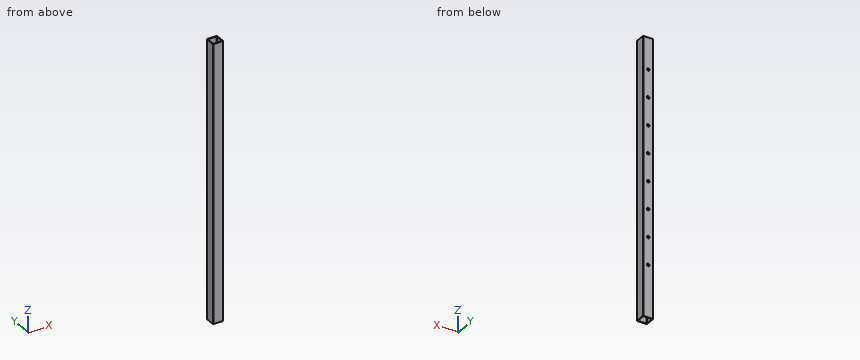
from build123d import *

# Parameters (mm, degrees)
SKETCH3_W           = 19.05
SKETCH3_H           = 19.05
SKETCH3_W_2         = 16.5608
SKETCH3_H_2         = 16.5608
BOSS_EXTRUDE1_DEPTH = 254.635
FILLET1_R           = 1.2446
CUT_EXTRUDE1_REACH  = 257.524
SKETCH4_R           = 2.413


with BuildPart() as part:
    # Sketch3 → Boss-Extrude1 (new, symmetric)
    with BuildSketch(Plane.XY):
        Rectangle(SKETCH3_W, SKETCH3_H)
        Rectangle(SKETCH3_W_2, SKETCH3_H_2, mode=Mode.SUBTRACT)
    extrude(amount=BOSS_EXTRUDE1_DEPTH, both=True)

    # Fillet1
    fillet1_edges = [part.edges().sort_by_distance(p)[0] for p in [
        (-8.2804, -8.2804, 0),
        (8.2804, -8.2804, 0),
        (8.2804, 8.2804, 0),
        (-8.2804, 8.2804, 0),
        (9.525, -9.525, 0),
        (-9.525, -9.525, 0),
        (-9.525, 9.525, 0),
        (9.525, 9.525, 0),
    ]]
    fillet(fillet1_edges, radius=FILLET1_R)

    # Sketch4 → Cut-Extrude1 (cut, up to next)
    with BuildSketch(Plane(origin=(0, 9.525, 0), x_dir=(1, 0, 0), z_dir=(0, 1, 0)), mode=Mode.PRIVATE) as cut_extrude1_sk1:
        with Locations(Location((0, 159.385, 0), (0, 0, 270))):
            Circle(SKETCH4_R)
    cut_extrude1_tool1 = extrude(cut_extrude1_sk1.sketch, amount=-CUT_EXTRUDE1_REACH, mode=Mode.PRIVATE) & part.part
    # Sketch4 → Cut-Extrude1 (cut, up to next)
    with BuildSketch(Plane(origin=(0, 9.525, 0), x_dir=(1, 0, 0), z_dir=(0, 1, 0)), mode=Mode.PRIVATE) as cut_extrude1_sk2:
        with Locations(Location((0, 108.585, 0), (0, 0, 270))):
            Circle(SKETCH4_R)
    cut_extrude1_tool2 = extrude(cut_extrude1_sk2.sketch, amount=-CUT_EXTRUDE1_REACH, mode=Mode.PRIVATE) & part.part
    # Sketch4 → Cut-Extrude1 (cut, up to next)
    with BuildSketch(Plane(origin=(0, 9.525, 0), x_dir=(1, 0, 0), z_dir=(0, 1, 0)), mode=Mode.PRIVATE) as cut_extrude1_sk3:
        with Locations(Location((0, 57.785, 0), (0, 0, 270))):
            Circle(SKETCH4_R)
    cut_extrude1_tool3 = extrude(cut_extrude1_sk3.sketch, amount=-CUT_EXTRUDE1_REACH, mode=Mode.PRIVATE) & part.part
    # Sketch4 → Cut-Extrude1 (cut, up to next)
    with BuildSketch(Plane(origin=(0, 9.525, 0), x_dir=(1, 0, 0), z_dir=(0, 1, 0)), mode=Mode.PRIVATE) as cut_extrude1_sk4:
        with Locations(Location((0, 6.985, 0), (0, 0, 270))):
            Circle(SKETCH4_R)
    cut_extrude1_tool4 = extrude(cut_extrude1_sk4.sketch, amount=-CUT_EXTRUDE1_REACH, mode=Mode.PRIVATE) & part.part
    # Sketch4 → Cut-Extrude1 (cut, up to next)
    with BuildSketch(Plane(origin=(0, 9.525, 0), x_dir=(1, 0, 0), z_dir=(0, 1, 0)), mode=Mode.PRIVATE) as cut_extrude1_sk5:
        with Locations(Location((0, -43.815, 0), (0, 0, 270))):
            Circle(SKETCH4_R)
    cut_extrude1_tool5 = extrude(cut_extrude1_sk5.sketch, amount=-CUT_EXTRUDE1_REACH, mode=Mode.PRIVATE) & part.part
    # Sketch4 → Cut-Extrude1 (cut, up to next)
    with BuildSketch(Plane(origin=(0, 9.525, 0), x_dir=(1, 0, 0), z_dir=(0, 1, 0)), mode=Mode.PRIVATE) as cut_extrude1_sk6:
        with Locations(Location((0, -94.615, 0), (0, 0, 270))):
            Circle(SKETCH4_R)
    cut_extrude1_tool6 = extrude(cut_extrude1_sk6.sketch, amount=-CUT_EXTRUDE1_REACH, mode=Mode.PRIVATE) & part.part
    # Sketch4 → Cut-Extrude1 (cut, up to next)
    with BuildSketch(Plane(origin=(0, 9.525, 0), x_dir=(1, 0, 0), z_dir=(0, 1, 0)), mode=Mode.PRIVATE) as cut_extrude1_sk7:
        with Locations(Location((0, -145.415, 0), (0, 0, 270))):
            Circle(SKETCH4_R)
    cut_extrude1_tool7 = extrude(cut_extrude1_sk7.sketch, amount=-CUT_EXTRUDE1_REACH, mode=Mode.PRIVATE) & part.part
    # Sketch4 → Cut-Extrude1 (cut, up to next)
    with BuildSketch(Plane(origin=(0, 9.525, 0), x_dir=(1, 0, 0), z_dir=(0, 1, 0)), mode=Mode.PRIVATE) as cut_extrude1_sk8:
        with Locations(Location((0, -196.215, 0), (0, 0, 270))):
            Circle(SKETCH4_R)
    cut_extrude1_tool8 = extrude(cut_extrude1_sk8.sketch, amount=-CUT_EXTRUDE1_REACH, mode=Mode.PRIVATE) & part.part
    add(cut_extrude1_tool1.solids().sort_by_distance((0, 9.525, -159.385))[0], mode=Mode.SUBTRACT)
    add(cut_extrude1_tool2.solids().sort_by_distance((0, 9.525, -108.585))[0], mode=Mode.SUBTRACT)
    add(cut_extrude1_tool3.solids().sort_by_distance((0, 9.525, -57.785))[0], mode=Mode.SUBTRACT)
    add(cut_extrude1_tool4.solids().sort_by_distance((0, 9.525, -6.985))[0], mode=Mode.SUBTRACT)
    add(cut_extrude1_tool5.solids().sort_by_distance((0, 9.525, 43.815))[0], mode=Mode.SUBTRACT)
    add(cut_extrude1_tool6.solids().sort_by_distance((0, 9.525, 94.615))[0], mode=Mode.SUBTRACT)
    add(cut_extrude1_tool7.solids().sort_by_distance((0, 9.525, 145.415))[0], mode=Mode.SUBTRACT)
    add(cut_extrude1_tool8.solids().sort_by_distance((0, 9.525, 196.215))[0], mode=Mode.SUBTRACT)


solid = part.part
CAD build for the part. Positions are in the model's coordinates, mm. Round coordinates to 2 decimals unless told otherwise and drop trailing zeros. Write each loop counter-clockwise with the first axis right and the second up, starting at its lowest first coordinate (ties: lowest second). Pieces come first, ordered by that corner, then holes. Notation, with made-up numbers: M 57.5,65.25 L 107.5,65.25 A29 cw 107.5,103.25 Z; hole C -15,5 d4. An arc over 180 degrees is marked long. Use a Markdown table: item, result. Add a question column.
1. Flat gauge pins, fed straight in: P1, Ø4.5, axis at x = 0, z = 43.815, coming from the +Y side; P2, Ø1.5, axis at x = -3.5, y = -7, coming from the -Z side. Where does each tip first touch, or does it go through?
2. Slice it at A-A on y = 2. Give the cut face in (x, z) (3 decimals).
3. Slice it at B-B on z = -39. Give the cut face in (x, y) (3 decimals), then the cut area to 3 significant figures.
4. Drill centre lines: probe 1 along Y at (x, z) = (6.25, -43.5) (3 decimals); probe 2 along Y at (x, z) = (7.5, 131) (3 decimals). Where is each one in solid material? Low to high.
Reply:
| question | item | result |
|---|---|---|
| 1 | P1 | stops at y = -8.28 |
| 1 | P2 | passes through |
| 2 | outline | M -9.525,-254.635 L -8.28,-254.635 L -8.28,254.635 L -9.525,254.635 Z; M 8.28,-254.635 L 9.525,-254.635 L 9.525,254.635 L 8.28,254.635 Z |
| 3 | outline | M -9.525,-8.28 A1.245 ccw -8.28,-9.525 L 8.28,-9.525 A1.245 ccw 9.525,-8.28 L 9.525,8.28 A1.245 ccw 8.28,9.525 L -8.28,9.525 A1.245 ccw -9.525,8.28 Z; hole M -8.28,-7.036 A1.245 ccw -7.036,-8.28 L 7.036,-8.28 A1.245 ccw 8.28,-7.036 L 8.28,7.036 A1.245 ccw 7.036,8.28 L -7.036,8.28 A1.245 ccw -8.28,7.036 Z |
| 3 | area | 88.6 mm^2 |
| 4 | probe 1 | y = -9.525 to -8.28, 8.28 to 9.525 |
| 4 | probe 2 | y = -9.525 to -8.191, 8.191 to 9.525 |
